Drawing for the job (mm, zero at the part's lowest x, y, z). Give positions to 0.01 mm unless a question says otherwise; leave off trailing zeros. Write each loop counter-clockwise with the first axis right and the second up, starting at its lowest first coordinate (ties: lowest second). Pieces come first, ordered by that corner, then holes.
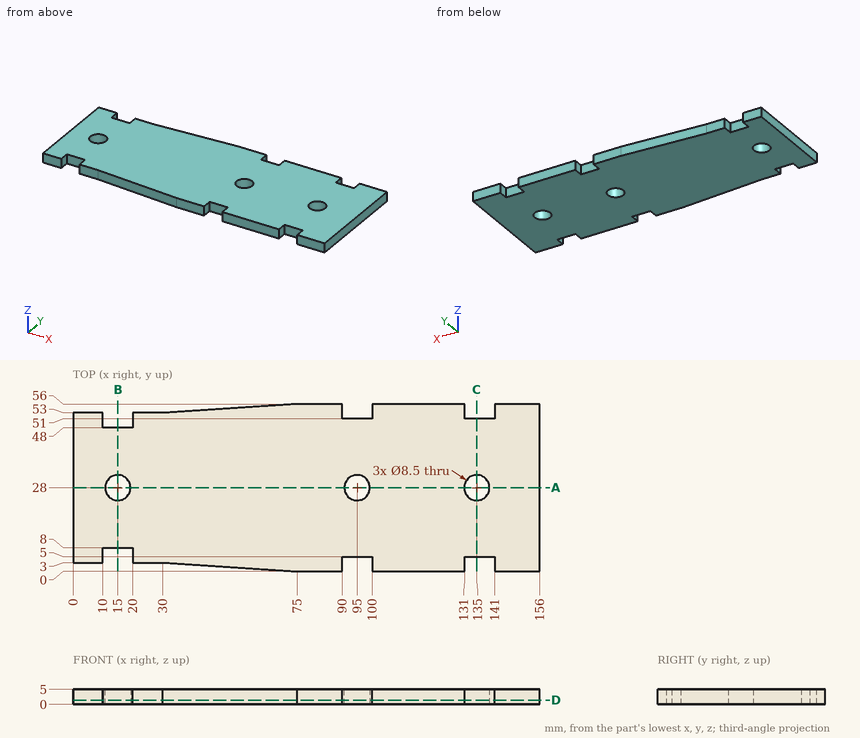
1. Slice it at B-B, the plane x = 15. Write the cut outline in (y, z).
Calculated:
outline: (8, 0) - (23.75, 0) - (23.75, 5) - (8, 5) - close; (32.25, 0) - (48, 0) - (48, 5) - (32.25, 5) - close
2. Slice it at D-D, the plane z = 1.45. State how many separate pieces and enclosed holes the cut face has, and give its area (3 significant figures).
Calculated:
separate pieces: 1
enclosed holes: 3
area: 7,950 mm2
3. Slice it at A-A, the plane y = 28. Write the cut outline in (x, z), and give its area (4 significant figures).
Calculated:
outline: (0, 0) - (10.75, 0) - (10.75, 5) - (0, 5) - close; (19.25, 0) - (90.75, 0) - (90.75, 5) - (19.25, 5) - close; (99.25, 0) - (130.75, 0) - (130.75, 5) - (99.25, 5) - close; (139.25, 0) - (156, 0) - (156, 5) - (139.25, 5) - close
area: 652.5 mm2
4. Slice it at C-C, the plane x = 135. Write the cut outline in (y, z).
Calculated:
outline: (5, 0) - (23.75, 0) - (23.75, 5) - (5, 5) - close; (32.25, 0) - (51, 0) - (51, 5) - (32.25, 5) - close
5. Probe probe 1 along X at (y, z) = (49, 4.15); probe 2 along X at (y, z) = (24.5, 1.1); probe 3 along Y at (x, z) = (29.5, 4.5). List the from-to ranges inside material, lowest first.
Calculated:
probe 1: x = 0 to 10, 20 to 156
probe 2: x = 0 to 12.59, 17.41 to 92.59, 97.41 to 132.59, 137.41 to 156
probe 3: y = 3 to 53
6. Pin check, flat tips, straight feed: P1, Ø2.5, axis at x = 96, z = 3, coming from the +Y side; P2, Ø1.5, axis at x = 26, z = 3, coming from the -Y side; P3, Ø2.5, axis at x = 136, z = 2.5, coming from the -Y side. Stop position of each tip, or through.
Calculated:
P1: stops at y = 51
P2: stops at y = 3
P3: stops at y = 5
